```python
from build123d import *

# Parameters (mm, degrees)
SKETCH1_W           = 9.6266
SKETCH1_H           = 8.3566
SKETCH1_R           = 2.2225
BOSS_EXTRUDE1_DEPTH = 2.54
SKETCH1_3_W         = 9.6266
SKETCH1_3_H         = 1.27
BOSS_EXTRUDE2_DEPTH = 20.32
CUT_EXTRUDE1_REACH  = 24.492
SKETCH2_R           = 2.2225
FILLET1_R           = 2.54


with BuildPart() as part:
    # Sketch1 → Boss-Extrude1 (new body)
    with BuildSketch(Plane(origin=(0, 0, 0), x_dir=(1, 0, 0), z_dir=(0, 1, 0))):
        with Locations((0, -0.635)):
            Rectangle(SKETCH1_W, SKETCH1_H)
        with Locations(Location((0, 0, 0), (0, 0, 270))):
            Circle(SKETCH1_R, mode=Mode.SUBTRACT)
    extrude(amount=BOSS_EXTRUDE1_DEPTH)

    # Sketch1_3 → Boss-Extrude2 (add)
    with BuildSketch(Plane(origin=(0, 0, 0), x_dir=(1, 0, 0), z_dir=(0, 1, 0))):
        with Locations((0, 4.1783)):
            Rectangle(SKETCH1_3_W, SKETCH1_3_H)
    extrude(amount=BOSS_EXTRUDE2_DEPTH)

    # Sketch2 → Cut-Extrude1 (cut, up to next)
    with BuildSketch(Plane.XY.offset(-3.5433), mode=Mode.PRIVATE) as cut_extrude1_sk1:
        with Locations((0, 15.24)):
            Circle(SKETCH2_R)
    cut_extrude1_tool1 = extrude(cut_extrude1_sk1.sketch, amount=-CUT_EXTRUDE1_REACH, mode=Mode.PRIVATE) & part.part
    add(cut_extrude1_tool1.solids().sort_by_distance((0, 15.24, -3.5433))[0], mode=Mode.SUBTRACT)

    # Fillet1
    fillet1_edges = [part.edges().sort_by_distance(p)[0] for p in [
        (0, 0, -4.8133),
    ]]
    fillet(fillet1_edges, radius=FILLET1_R)


solid = part.part
```
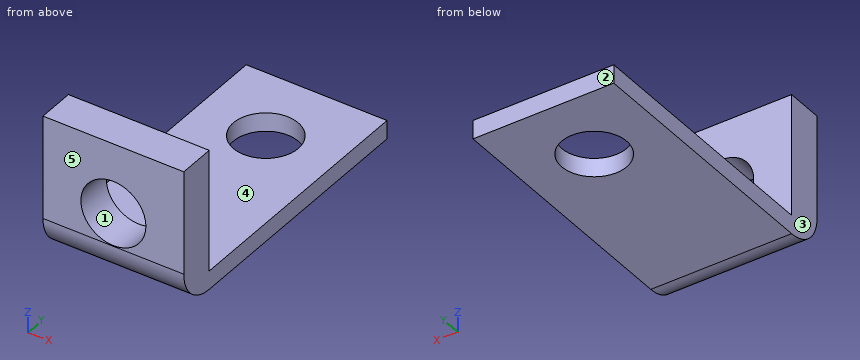
Can you work these out from the model? Positions are in its coordinate system, mm. Face numbers are marked on the shaded views. A direction names the side the tool comes from. Coordinates: 2 decimals unless noted, no trailing zeros. Loops run counter-clockwise (first coordinate to the right, second up) from the corner with the lowest first, then second, coordinate; pieces in that order, holes last. Notation, with made-up numbers: (0, 19) -> (31, 19) arc R24 ccw to (31, 56) -> close; hole circle Ø1 at (-6, 4.5). An arc over 180 degrees is marked (long way). Answer as a JSON object with one key per item and string values.
1) If I drill on line 1 (X direction, y = 2, z = 0); line 2 (Y direction, x = -2.5, z = -0.5); line 3 (Z direction, x = 0, y = 5.5), over which ranges is the centre line in solid material (lowest first)?
Results:
{"line 1": "x = -4.81 to -2.22, 2.22 to 4.81", "line 2": "y = 0 to 2.54", "line 3": "z = -4.81 to -3.54"}
2) Imagine slicing it at D-D (x = 3.5). Please give me the cut outline in (y, z).
Results:
{"outline": "(0, -2.27) arc R2.54 ccw to (2.54, -4.81) -> (20.32, -4.81) -> (20.32, -3.54) -> (2.54, -3.54) -> (2.54, 4.81) -> (0, 4.81) -> close"}
3) For P1, Ø1, axis at x = -2.5, z = -1, coming from the +Y side, with a flat end and sliding along its axis, tell me the tip position at first contact or that it passes through.
Results:
{"P1": "stops at y = 2.54"}
4) Thinking about a two-plate mould opening in X: for the marked faces 1, 2 and 3, which applies, pulls with the +X half, pulls with the -X half, needs draft (parallel to the pull), parting line crosses it, or undercut?
Results:
{"face 1": "undercut", "face 2": "needs draft", "face 3": "pulls with the -X half"}
5) Imagine slicing it at B-B (z = 0). Please give me the cut outline in (x, y), then the cut area to 3 significant figures.
Results:
{"outline": "(-4.81, 0) -> (-2.22, 0) -> (-2.22, 2.54) -> (-4.81, 2.54) -> close; (2.22, 0) -> (4.81, 0) -> (4.81, 2.54) -> (2.22, 2.54) -> close", "area": "13.2 mm^2"}
6) For the marked faces 4 and 5, which set-ups out of +Z, -Z, +X, -X, +Y, -Y let a thin tool reach every point of the face, with its end or its side?
Results:
{"face 4": "+Z, +X, -X, +Y", "face 5": "+Z, -Z, +X, -X, -Y"}
7) Imagine slicing it at A-A (y = 15.24). Please give me the cut outline in (x, z), then the cut area to 3 significant figures.
Results:
{"outline": "(-4.81, -4.81) -> (-2.22, -4.81) -> (-2.22, -3.54) -> (-4.81, -3.54) -> close; (2.22, -4.81) -> (4.81, -4.81) -> (4.81, -3.54) -> (2.22, -3.54) -> close", "area": "6.58 mm^2"}
8) Imagine slicing it at C-C (x = 0). Please give me the cut outline in (y, z), then the cut area to 3 significant figures.
Results:
{"outline": "(0, -2.27) arc R2.54 ccw to (2.54, -4.81) -> (13.02, -4.81) -> (13.02, -3.54) -> (2.54, -3.54) -> (2.54, -2.22) -> (0, -2.22) -> close; (0, 2.22) -> (2.54, 2.22) -> (2.54, 4.81) -> (0, 4.81) -> close; (17.46, -4.81) -> (20.32, -4.81) -> (20.32, -3.54) -> (17.46, -3.54) -> close", "area": "28.7 mm^2"}
